The model under review builds one solid part; all positions refer to its coordinate system, in mm. A direction names the side the tool comes from. Give positions to 0.01 mm unless a question says otherwise; leave off trailing zeros. Loops run counter-clockwise (first coordinate to the right, second up) from the corner with the lowest first, then second, coordinate; pieces in that order, holes last. Notation, with made-up numbers: M 86.25,-14 L 103.25,-14 A14 ccw 103.25,4 Z; hole C 35,36 d3. An arc over 180 degrees is marked long. Return JSON: item names as keys, results as strings. Group by question number.
```python
from build123d import *

# Parameters (mm, degrees)
SKETCH1_W           = 0.8999999999999999
SKETCH1_H           = 5.9
BOSS_EXTRUDE1_DEPTH = 30
SKETCH1_3_R         = 3
SKETCH1_3_W         = 0.8999999999999999
SKETCH1_3_H         = 5.9
BOSS_EXTRUDE2_DEPTH = 21.51
SKETCH1_4_R         = 5.35
SKETCH1_4_R_2       = 3
BOSS_EXTRUDE3_DEPTH = 21.5
SKETCH1_5_R         = 5.35
BOSS_EXTRUDE4_DEPTH = 17
BOSS_EXTRUDE5_DEPTH = 3.1
SKETCH2_R           = 4.5
SKETCH2_R_2         = 3
CUT_EXTRUDE1_DEPTH  = 19.5
SKETCH3_R           = 2.175
CUT_EXTRUDE2_DEPTH  = 4.1
SKETCH4_R           = 2.1
CUT_EXTRUDE3_DEPTH  = 15.9
SKETCH5_R           = 0.9000000000000007
CUT_EXTRUDE4_DEPTH  = 32.693887423287165
FILLET1_R           = 0.5


with BuildPart() as part:
    # Sketch1 → Boss-Extrude1 (new body)
    with BuildSketch(Plane(origin=(0, 0, 0), x_dir=(1, 0, 0), z_dir=(0, 1, 0))):
        Rectangle(SKETCH1_W, SKETCH1_H)
    extrude(amount=-BOSS_EXTRUDE1_DEPTH)

    # Sketch1_3 → Boss-Extrude2 (add)
    with BuildSketch(Plane(origin=(0, 0, 0), x_dir=(1, 0, 0), z_dir=(0, 1, 0))):
        with Locations(Location((5.2e-15, -1.388e-14, 0), (0, 0, 270))):
            Circle(SKETCH1_3_R)
        Rectangle(SKETCH1_3_W, SKETCH1_3_H)
    extrude(amount=-BOSS_EXTRUDE2_DEPTH)

    # Sketch1_4 → Boss-Extrude3 (add)
    with BuildSketch(Plane(origin=(0, 0, 0), x_dir=(1, 0, 0), z_dir=(0, 1, 0))):
        with Locations(Location((5.2e-15, -1.388e-14, 0), (0, 0, 270))):
            Circle(SKETCH1_4_R)
        with Locations(Location((5.2e-15, -1.388e-14, 0), (0, 0, 270))):
            Circle(SKETCH1_4_R_2, mode=Mode.SUBTRACT)
    extrude(amount=-BOSS_EXTRUDE3_DEPTH)

    # Sketch1_5 → Boss-Extrude4 (add)
    with BuildSketch(Plane(origin=(0, 0, 0), x_dir=(1, 0, 0), z_dir=(0, 1, 0))):
        with BuildLine():
            ThreePointArc((-5.365000000000034, -2.4549490829749705), (-2.3169e-13, -5.900000000000015), (5.3649999999998474, -2.4549490829754013))
            Line((5.365000000000007, -2.454949082975432), (5.365000000000007, 2.4549490829754035))
            ThreePointArc((5.364999999999848, 2.454949082975371), (-2.2894e-13, 5.899999999999986), (-5.365000000000033, 2.4549490829749443))
            Line((-5.364999999999993, 2.4549490829749345), (-5.364999999999993, -2.454949082974963))
        make_face()
        with Locations(Location((5.2e-15, -1.388e-14, 0), (0, 0, 270))):
            Circle(SKETCH1_5_R, mode=Mode.SUBTRACT)
    extrude(amount=-BOSS_EXTRUDE4_DEPTH)

    # Sketch1_6 → Boss-Extrude5 (add)
    with BuildSketch(Plane(origin=(0, 0, 0), x_dir=(1, 0, 0), z_dir=(0, 1, 0))):
        with BuildLine():
            ThreePointArc((-5.364999999999868, -4.496306817822988), (4.744e-14, -7.000000000000014), (5.364999999999932, -4.4963068178229255))
            Line((5.365000000000007, -4.496306817822948), (5.365000000000007, -2.454949082975432))
            ThreePointArc((5.3649999999998474, -2.4549490829754013), (-2.3169e-13, -5.900000000000015), (-5.365000000000034, -2.4549490829749705))
            Line((-5.364999999999993, -2.454949082974963), (-5.364999999999993, -4.496306817823026))
        make_face()
        with BuildLine():
            ThreePointArc((5.364999999999927, 4.4963068178229015), (4.294e-14, 6.999999999999986), (-5.364999999999867, 4.496306817822961))
            Line((-5.364999999999993, 4.4963068178229975), (-5.364999999999993, 2.4549490829749345))
            ThreePointArc((-5.365000000000033, 2.4549490829749443), (-2.2894e-13, 5.899999999999986), (5.364999999999848, 2.454949082975371))
            Line((5.365000000000007, 2.4549490829754035), (5.365000000000007, 4.496306817822926))
        make_face()
        with BuildLine():
            ThreePointArc((-5.365000000000033, 2.4549490829749443), (-5.899999999999995, -1.316e-14), (-5.365000000000034, -2.4549490829749705))
            Line((-5.364999999999993, -2.454949082974963), (-5.364999999999993, 2.4549490829749345))
        make_face()
        with BuildLine():
            ThreePointArc((-5.364999999999867, 4.496306817822961), (-6.999999999999995, -1.302e-14), (-5.364999999999867, -4.49630681782299))
            Line((-5.364999999999993, -4.496306817823026), (-5.364999999999993, -2.454949082974963))
            ThreePointArc((-5.365000000000034, -2.4549490829749705), (-5.899999999999995, -1.316e-14), (-5.365000000000033, 2.4549490829749443))
            Line((-5.364999999999993, 2.4549490829749345), (-5.364999999999993, 4.4963068178229975))
        make_face()
        with BuildLine():
            Line((5.365000000000007, -2.454949082975432), (5.365000000000007, -4.496306817822948))
            ThreePointArc((5.364999999999932, -4.4963068178229255), (6.578563673021629, -2.392174742781203), (7.000000000000005, -1.559e-14))
            ThreePointArc((7.000000000000005, -1.388e-14), (6.578563673021627, 2.3921747427811804), (5.364999999999927, 4.4963068178229015))
            Line((5.365000000000007, 4.496306817822926), (5.365000000000007, 2.4549490829754035))
            ThreePointArc((5.364999999999848, 2.4549490829753706), (5.7646986044371475, 1.2562842035146455), (5.900000000000006, -1.388e-14))
            ThreePointArc((5.900000000000006, -1.532e-14), (5.7646986044371475, -1.2562842035146757), (5.3649999999998474, -2.4549490829754013))
        make_face()
        with BuildLine():
            Line((5.365000000000007, 2.4549490829754035), (5.365000000000007, -2.454949082975432))
            ThreePointArc((5.3649999999998474, -2.4549490829754013), (5.7646986044371475, -1.2562842035146757), (5.900000000000006, -1.532e-14))
            ThreePointArc((5.900000000000006, -1.388e-14), (5.7646986044371475, 1.2562842035146455), (5.364999999999848, 2.4549490829753706))
        make_face()
    extrude(amount=-BOSS_EXTRUDE5_DEPTH)

    # Sketch2 → Cut-Extrude1 (cut)
    with BuildSketch(Plane(origin=(0, 0, 0), x_dir=(1, 0, 0), z_dir=(0, 1, 0))):
        with Locations(Location((0, 0, 0), (0, 0, 270))):
            Circle(SKETCH2_R)
        with Locations(Location((0, 0, 0), (0, 0, 270))):
            Circle(SKETCH2_R_2, mode=Mode.SUBTRACT)
    extrude(amount=-CUT_EXTRUDE1_DEPTH, mode=Mode.SUBTRACT)

    # Sketch3 → Cut-Extrude2 (cut)
    with BuildSketch(Plane(origin=(0, 0, 0), x_dir=(1, 0, 0), z_dir=(0, 1, 0))):
        with Locations(Location((0, 0, 0), (0, 0, 270))):
            Circle(SKETCH3_R)
    extrude(amount=-CUT_EXTRUDE2_DEPTH, mode=Mode.SUBTRACT)

    # Sketch4 → Cut-Extrude3 (cut)
    with BuildSketch(Plane(origin=(0, -4.1, 0), x_dir=(1, 0, 0), z_dir=(0, 1, 0))):
        with Locations(Location((0, 0, 0), (0, 0, 270))):
            Circle(SKETCH4_R)
    extrude(amount=-CUT_EXTRUDE3_DEPTH, mode=Mode.SUBTRACT)

    # Sketch5 → Cut-Extrude4 (cut, through all)
    with BuildSketch(Plane.ZY.offset(0.4499999999999899)):
        with Locations((4.3e-16, -26.099999999999998)):
            Circle(SKETCH5_R)
    extrude(amount=-CUT_EXTRUDE4_DEPTH, mode=Mode.SUBTRACT)

    # Fillet1
    fillet1_edges = [part.edges().sort_by_distance(p)[0] for p in [
        (1.005e-14, -30, -2.9500000000000126),
        (1.01e-14, -30, 2.949999999999988),
        (-5.3649999999999185, 0, -4.496306817822891),
        (1.38e-15, 0, -4.5),
        (9.2e-16, 0, -3),
    ]]
    fillet(fillet1_edges, radius=FILLET1_R)


solid = part.part
```
(1) Add section A-A (y = -10.5). Write out the cut boundary in (x, z) (3 decimals), and give its area (3 significant figures).
(2) For probe 1 along X at (y, z) = (-7.25, 0) (3 decimals); probe 2 along X at (y, z) = (-17.25, 0); probe 3 along Y at (x, z) = (0.2, 0), list the stretches that pass through material, from the lowest coordinate up.
(3) Mouldability with a two-part tool opening along Z and no side actions: class faces 5 (the flat face through (0, -25, -2.95)), 6 (the flat face through (0, -20, 0)), 7 (the flat face through (0.45, -25, 0)) as released by +Z, released by -Z, zero draft, split by the parting line, or undercut.
(4) Add section B-B (y = -26.1). Write out the cut boundary in (x, z), and give its area (3 significant figures).
(5) For pin 1 (1.8 mm diameter, centred on y = -27.5, z = -1, fed in from -X); pin 2 (1.8 mm diameter, centred on y = -24.5, z = -1, fed in from +X); pin 3 (1 mm diameter, centred on x = 2.5, y = -7.5, fed in from +Z), all flat-tipped, find the tip position at first contact; note any pin that passes through.
(6) For faces 1 (the flat face through (-5.365, -10, 0)), 2 (the flat face through (6, -3.1, -1)), 3 (the flat face through (0, -25, 2.95)), 4 (the flat face through (-3, -19.5, 1)), list the 3-axis set-ups (+Z, -Z, +X, -X, +Y, -Y) from which the entire face can be reached by the end or side of a thin tool; tool diameter is ignored.
(7) Add section C-C (y = -19). Write out the cut boundary in (x, z), and give its area (3 significant figures).
Verdict:
{
 "1": {"outline": "M -5.365,-2.455 A5.9 ccw 5.365,-2.455 L 5.365,2.455 A5.9 ccw -5.365,2.455 Z; C 0,0 d6; hole C 0,0 d9; hole C 0,0 d4.2", "area": "56.6 mm²"},
 "2": {"probe 1": "x = -5.365 to -4.5, -3 to -2.1, 2.1 to 3, 4.5 to 5.365", "probe 2": "x = -5.35 to -4.5, -3 to -2.1, 2.1 to 3, 4.5 to 5.35", "probe 3": "y = -30 to -27, -25.2 to -20"},
 "3": {"face 5": "released by -Z", "face 6": "undercut", "face 7": "zero draft"},
 "4": {"outline": "M -0.45,-2.95 L 0.45,-2.95 L 0.45,-0.9 L -0.45,-0.9 Z; M -0.45,0.9 L 0.45,0.9 L 0.45,2.95 L -0.45,2.95 Z", "area": "3.69 mm²"},
 "5": {"pin 1": "stops at x = -0.45", "pin 2": "stops at x = 0.45", "pin 3": "stops at z = 5.55"},
 "6": {"face 1": "+Z, -Z, -X, -Y", "face 2": "-Y", "face 3": "+Z, +X, -X, -Y", "face 4": "+Y"},
 "7": {"outline": "C 0,0 d10.7; C 0,0 d6; hole C 0,0 d9; hole C 0,0 d4.2", "area": "40.7 mm²"}
}
